Build history of the part. All positions in model axes, mm. A direction names the side the tool comes from. Round coordinates to 2 decimals unless told otherwise and drop trailing zeros. Write each loop counter-clockwise with the first axis right and the second up, starting at its lowest first coordinate (ties: lowest second). Pieces come first, ordered by that corner, then holes. Notation, with made-up numbers: (-38.5, 28) -> (-9.5, 28) arc R20 ccw to (-9.5, 53) -> close; hole circle Ø11 at (-21.5, -35). An arc over 180 degrees is marked (long way). Answer as CSV lines item,"result".
from build123d import *

# Parameters (mm, degrees)
SKETCH2_R           = 15
SKETCH2_R_2         = 11
BOSS_EXTRUDE1_DEPTH = 4
SKETCH3_R           = 15
SKETCH3_R_2         = 4
BOSS_EXTRUDE2_DEPTH = 8
BOSS_EXTRUDE5_DEPTH = 12
BOSS_EXTRUDE7_DEPTH = 8
SKETCH9_R           = 2.875
CUT_EXTRUDE1_DEPTH  = 14


with BuildPart() as part:
    # Sketch2 → Boss-Extrude1 (new body)
    with BuildSketch(Plane.XY):
        Circle(SKETCH2_R)
        Circle(SKETCH2_R_2, mode=Mode.SUBTRACT)
    extrude(amount=BOSS_EXTRUDE1_DEPTH)

    # Sketch3 → Boss-Extrude2 (add)
    with BuildSketch(Plane.XY.offset(4)):
        Circle(SKETCH3_R)
        Circle(SKETCH3_R_2, mode=Mode.SUBTRACT)
    extrude(amount=BOSS_EXTRUDE2_DEPTH)

    # Sketch6 → Boss-Extrude5 (add)
    with BuildSketch(Plane.XY.offset(12)):
        with BuildLine():
            Line((-15, 0), (-15, -33))
            Line((-15, -33), (15, -33))
            Line((15, -33), (15, 0))
            ThreePointArc((15, 0), (0, -15), (-15, 0))
        make_face()
    extrude(amount=-BOSS_EXTRUDE5_DEPTH)

    # Sketch8 → Boss-Extrude7 (add)
    with BuildSketch(Plane.XY.offset(12)):
        with BuildLine():
            Line((-3.013818176, 2.63), (-3.013818176, -2.63))
            ThreePointArc((-3.013818176, -2.63), (-4, 0), (-3.013818176, 2.63))
        make_face()
    extrude(amount=-BOSS_EXTRUDE7_DEPTH)

    # Sketch9 → Cut-Extrude1 (cut)
    with BuildSketch(Plane.XZ.offset(33)):
        with Locations((-7, 6)):
            Circle(SKETCH9_R)
        with Locations((7, 6)):
            Circle(SKETCH9_R)
    extrude(amount=-CUT_EXTRUDE1_DEPTH, mode=Mode.SUBTRACT)


solid = part.part
1. Cut at A-A, the plane x = 0. Write the cut outline in (y, z).
Results found:
outline,"(-33, 0) -> (-11, 0) -> (-11, 4) -> (-4, 4) -> (-4, 12) -> (-33, 12) -> close; (4, 4) -> (11, 4) -> (11, 0) -> (15, 0) -> (15, 12) -> (4, 12) -> close"
2. Cut at D-D, the plane x = -8.75. Write the cut outline in (y, z).
Results found:
outline,"(-33, 0) -> (-6.67, 0) -> (-6.67, 4) -> (6.67, 4) -> (6.67, 0) -> (12.18, 0) -> (12.18, 12) -> (-33, 12) -> (-33, 8.28) -> (-19, 8.28) -> (-19, 3.72) -> (-33, 3.72) -> close"
3. Cut at B-B, the plane z = 9.5. Write the cut outline in (x, y).
Results found:
outline,"(-15, -33) -> (15, -33) -> (15, 0) arc R15 ccw to (-15, 0) -> close; hole (-3.01, -2.63) arc R4 ccw (long way) to (-3.01, 2.63) -> close"
4. Mould opens along X. For faces 1 (the flat face through (-15, -16, 6)), 2 (the cylindrical face through (6.63, -26.1, 8.85)), 3 (the flat face through (0, -14, 0)) say: +X half, -X half, draft (parallel to the pull), parting line (faces both ways), or undercut.
Results found:
face 1,"-X half"
face 2,"undercut"
face 3,"draft"
5. Drop flat-ended pins along their axis: pin 1 Ø3 at (x, z) = (-2.5, 2) entering from +Y; pin 2 Ø3 at (x, z) = (7, 5) entering from -Y; pin 3 Ø3 at (x, z) = (-4.5, 1) entering from +Y. Give the stop position or say it passes through.
Results found:
pin 1,"stops at y = 14.97"
pin 2,"stops at y = -19"
pin 3,"stops at y = 14.7"
6. Cut at C-C, the plane y = -0.5. Write the cut outline in (x, z).
Results found:
outline,"(-15, 0) -> (-10.99, 0) -> (-10.99, 4) -> (-3.01, 4) -> (-3.01, 12) -> (-15, 12) -> close; (3.97, 4) -> (10.99, 4) -> (10.99, 0) -> (15, 0) -> (15, 12) -> (3.97, 12) -> close"
7. Probe line 1 along Y through (x, z) = (0, 6); line 2 along Z through (x, y) = (2.75, -10); line 3 along Z through (x, y) = (-7, -28.5) (3 decimals). List the from-to ranges inside material, lowest first.
Results found:
line 1,"y = -33 to -4, 4 to 15"
line 2,"z = 4 to 12"
line 3,"z = 0 to 3.125, 8.875 to 12"
8. Which spindle directions (+Z, -Z, +X, -X, +Y, -Y) get a long thin tool onto all of the face, cutting with end or side? Do faces 4 (the flat face through (-3.014, 0, 8)), 5 (the flat face through (0, -33, 6)), 6 (the cylindrical face through (-9.12, -26.1, 7.94)), 7 (the cylindrical face through (-2.38, -10.74, 1.97)), 8 (the flat face through (15, -17, 6)). Say none if no direction does.
Results found:
face 4,"+Z, -Z"
face 5,"+Z, -Z, +X, -X, -Y"
face 6,"-Y"
face 7,"-Z"
face 8,"+Z, -Z, +X, +Y, -Y"
